Design review of the part built by this model. Coordinates are the model's own, in mm. Face numbers are marked on the shaded views. A direction names the side the tool comes from. Give positions to 0.01 mm unless a question says otherwise; leave off trailing zeros. Write each loop counter-clockwise with the first axis right and the second up, starting at its lowest first coordinate (ties: lowest second). Pieces come first, ordered by that corner, then holes. Notation, with made-up numbers: M -2.5,87 L 6.5,87 A18 ccw 6.5,120 Z; hole C 47,-18.5 d1. An arc over 180 degrees is marked long. Use one line per item in the form item = value. Start each with the question number.
from build123d import *

# Parameters (mm, degrees)
F0_W     = 19.05
F0_H     = 19.05
F0_W_2   = 15.875
F0_H_2   = 15.875
F1_DEPTH = 140
F3_DEPTH = 9.526
F4_DEPTH = 9.526


with BuildPart() as f1:
    # F0 (on Front) → F1 (new body)
    with BuildSketch(Plane.XZ):
        Rectangle(F0_W, F0_H)
        Rectangle(F0_W_2, F0_H_2, mode=Mode.SUBTRACT)
    extrude(amount=F1_DEPTH)

    # F2 (on Top) → F3 (cut, through all)
    with BuildSketch(Plane.XY):
        Polygon((9.525, 0), (-9.525, 0), (-9.525, -19.05), align=None)
        Polygon((-9.525, -120.95), (-9.525, -140), (9.525, -140), align=None)
    extrude(amount=-F3_DEPTH, mode=Mode.SUBTRACT)

    # F2 (on Top) → F4 (cut, through all)
    with BuildSketch(Plane.XY):
        Polygon((9.525, 0), (-9.525, 0), (-9.525, -19.05), align=None)
        Polygon((-9.525, -120.95), (-9.525, -140), (9.525, -140), align=None)
    extrude(amount=F4_DEPTH, mode=Mode.SUBTRACT)


solid = f1.part
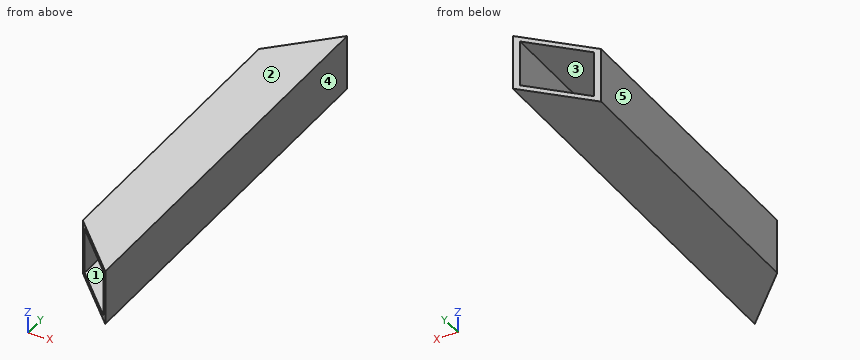
1. Clearance check with a flat-ended pin moving along its axis: pin 1 Ø6 at (x, z) = (-6.5, 2.5) entering from -Y. State where the tip first meets the part, or that it passes through.
2. We need section C-C (x = 0.25). State the section outline as (y, z) points (1 decimal), and give its area (3 significant figures).
3. We need section B-B (y = -83). State the section outline as (x, z) points (1 decimal), and give its area (3 significant figures).
4. To check wall thickness, follow L1, parallel to X at y = -19.5, z = 7.75 (1 decimal); L2, parallel to X at y = -11.5, z = 0.25 (1 decimal). State the ranges of each line that lie inside material, in increasing order.
5. We need section D-D (y = -13). State the section outline as (x, z) points (1 decimal), and give its area (3 significant figures).
6. For the marked faces 1 and 2, list the 3-axis set-ups (+Z, -Z, +X, -X, +Y, -Y) from which the entire face can be reached by the end or side of a thin tool; tool diameter is ignored.
7. Draft analysis for pull direction X (two halves, no side actions). For the marked faces 3, 4 and 5, state which applies: pulls with the +X half, pulls with the -X half, needs draft (parallel to the pull), parting line crosses it, or undercut.
Answer block:
q1.pin_1 = -122.54
q2.outline = M -130.7,-9.5 L -9.3,-9.5 L -9.3,-7.9 L -130.7,-7.9 Z; M -130.7,7.9 L -9.3,7.9 L -9.3,9.5 L -130.7,9.5 Z
q2.area = 386 mm^2
q3.outline = M -9.5,-9.5 L 9.5,-9.5 L 9.5,9.5 L -9.5,9.5 Z; hole M -7.9,-7.9 L 7.9,-7.9 L 7.9,7.9 L -7.9,7.9 Z
q3.area = 111 mm^2
q4.L1 = -9.5 to -7.9, 7.9 to 9.5
q4.L2 = 7.9 to 9.5
q5.outline = M -3.5,-9.5 L 9.5,-9.5 L 9.5,9.5 L -3.5,9.5 L -3.5,7.9 L 7.9,7.9 L 7.9,-7.9 L -3.5,-7.9 Z
q5.area = 66.5 mm^2
q6.face_1 = +Y, -Y
q6.face_2 = +Z, +X, -X, +Y, -Y
q7.face_3 = undercut
q7.face_4 = pulls with the +X half
q7.face_5 = pulls with the -X half
